Design review of the part built by this model. Coordinates are the model's own, in mm. A direction names the side the tool comes from. Coordinates: 2 decimals unless noted, no trailing zeros. Write each loop counter-clockwise with the first axis right and the second up, starting at its lowest first coordinate (ties: lowest second). Pieces come first, ordered by that corner, then holes. Notation, with made-up numbers: (57.25, 84) -> (102.25, 84) arc R6 ccw to (102.25, 92) -> close; hole circle Ø5 at (-13.75, -2). An arc over 180 degrees is marked (long way). Write item = value, one per line. Start each with the question number.
```python
from build123d import *

# Parameters (mm, degrees)
F0_R     = 5.08
F1_DEPTH = 22.86
F3_D     = 6.35
F4_R     = 4.863365
F5_DEPTH = 7.62
F7_D     = 6.096


with BuildPart() as f1:
    # F0 (on Top) → F1 (new body)
    with BuildSketch(Plane.XY):
        Circle(F0_R)
    extrude(amount=F1_DEPTH)

    # F3 (through all)
    with Locations(Plane(origin=(0, 0, 0), x_dir=(1, 0, 0), z_dir=(0, 0, -1))):
        with Locations((0, 0)):
            Hole(F3_D / 2)

    # F4 (on Right) → F5 (join)
    with BuildSketch(Plane.YZ):
        with Locations((0, 11.58422)):
            Circle(F4_R)
    extrude(amount=F5_DEPTH)

    # F7 (through all)
    with Locations(Plane.YZ.offset(7.62)):
        with Locations((0, 11.58422)):
            Hole(F7_D / 2)


solid = f1.part
```
(1) For line 1 (Y direction, x = 0, z = 17.5) (3 decimals); line 2 (Y direction, x = -2.5, z = 8.5); line 3 (Z direction, x = 2, y = 1), list the stretches that pass through material, from the lowest coordinate up.
(2) For pin 1 Ø1 at (y, z) = (-1.5, 5) entering from -X; pin 2 Ø4 at (y, z) = (2.5, 15.5) entering from -X; pin 3 Ø1.5 at (x, z) = (3.5, 17) entering from -Y; pin 4 Ø5 at (x, z) = (-2.5, 18) entering from +Y, all flat-tipped, find the tip position at first contact; note any pin that passes through.
(3) Take a section at D-D, the plane x = 4.25. State the section outline as (y, z) points.
(4) Take a section at B-B, the plane z = 13. State the section outline as (x, y) points (3 decimals).
(5) For faces 1 (the face through (0, -3, 13)), 2 (the face through (5.18, 2.61, 15.69)), 3 (the face through (-3.744, 3.433, 11.27)), 4 (the face through (3.3, -1.1, 0)), list the 3-axis set-ups (+Z, -Z, +X, -X, +Y, -Y) from which the entire face can be reached by the end or side of a thin tool; tool diameter is ignored.
(6) Mouldability with a two-part tool opening along X and no side actions: class faces 5 (the face through (3.757, 0.397, 14.606)), 6 (the face through (7.62, -2, 9)), 7 (the face through (-1.707, -2.677, 14.13)) as pulls with the +X half, pulls with the -X half, needs draft (parallel to the pull), parting line crosses it, or undercut.
(7) Take a section at A-A, the plane y = 0. State the section outline as (x, z) points (3 decimals).
(8) Take a section at C-C, the plane x = -2.5. State the section outline as (y, z) points, then the cut area to 3 significant figures.
Report:
q1.line_1 = -5.08 to -3.175, 3.175 to 5.08
q1.line_2 = -4.42 to -1.96, 1.96 to 4.42
q1.line_3 = 6.82 to 8.7, 14.46 to 16.34
q2.pin_1 = -4.98
q2.pin_2 = -5.06
q2.pin_3 = -4.27
q2.pin_4 = 5.08
q3.outline = (-2.78, 0) -> (2.78, 0) -> (2.78, 7.6) arc R4.86 ccw to (2.78, 15.57) -> (2.78, 22.86) -> (-2.78, 22.86) -> (-2.78, 15.57) arc R4.86 ccw to (-2.78, 7.6) -> close; hole circle Ø6.1 at (0, 11.58)
q4.outline = (-4.304, -2.699) arc R5.08 ccw to (2.039, -4.653) -> (7.62, -4.653) -> (7.62, -2.699) -> (0, -2.699) -> (0, -3.175) arc R3.175 cw to (-1.672, -2.699) -> close; (-4.304, 2.699) -> (-1.672, 2.699) arc R3.175 cw to (0, 3.175) -> (0, 2.699) -> (7.62, 2.699) -> (7.62, 4.653) -> (2.039, 4.653) arc R5.08 ccw to start
q5.face_1 = +Z, -Z
q5.face_2 = +X
q5.face_3 = none
q5.face_4 = -Z, +X, -X, +Y, -Y
q6.face_5 = needs draft
q6.face_6 = pulls with the +X half
q6.face_7 = undercut
q7.outline = (-5.08, 0) -> (-3.175, 0) -> (-3.175, 8.536) -> (-5.08, 8.536) -> close; (-5.08, 14.632) -> (-3.175, 14.632) -> (-3.175, 22.86) -> (-5.08, 22.86) -> close; (0, 6.721) -> (3.175, 6.721) -> (3.175, 0) -> (5.08, 0) -> (5.08, 6.721) -> (7.62, 6.721) -> (7.62, 8.536) -> (0, 8.536) -> close; (0, 14.632) -> (7.62, 14.632) -> (7.62, 16.448) -> (5.08, 16.448) -> (5.08, 22.86) -> (3.175, 22.86) -> (3.175, 16.448) -> (0, 16.448) -> close
q8.outline = (-4.42, 0) -> (-1.96, 0) -> (-1.96, 9.25) arc R3.05 cw to (-1.96, 13.92) -> (-1.96, 22.86) -> (-4.42, 22.86) -> close; (1.96, 0) -> (4.42, 0) -> (4.42, 22.86) -> (1.96, 22.86) -> (1.96, 13.92) arc R3.05 cw to (1.96, 9.25) -> close
q8.area = 106 mm2
